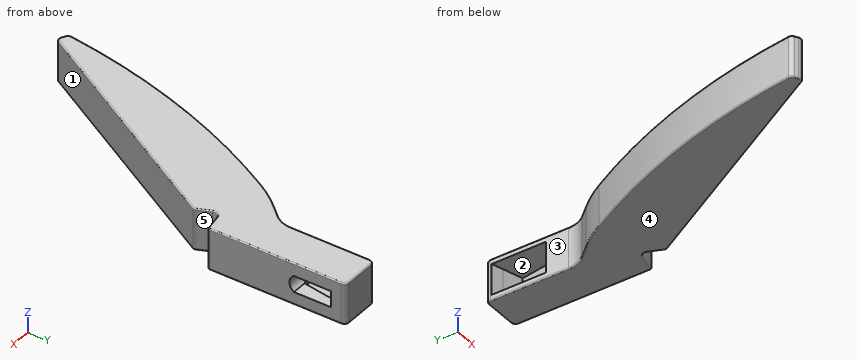
Autodesk Fusion 360 part; units mm, degrees
sketch "Sketch1" plane through (0, 0, 0) normal (1, 0, 0) x (0, 1, 0) in component "MitiVac Handle"
  line L0 (0, 0) -> (0, 3.5)
  line L1 (0, 3.5) -> (53.5, 3.5)
  line L2 (53.5, 3.5) -> (53.5, 0)
  line L3 (53.5, 0) -> (37.5, 0)
  line L4 (37.5, 0) -> (35.5, 0)
  line L5 (37.5, 0) -> (37.5, 3.5)
  line L6 (0, 0) -> (0, -3.5)
  line L7 (0, -3.5) -> (53.5, -3.5)
  line L8 (53.5, -3.5) -> (53.5, 0)
  line L9 (37.5, 0) -> (37.5, -3.5)
  arc A0 (37.5, 3.5) -> (37.5, -3.5) centre (39.5625, 0) ccw
  line L10 (0, 0) -> (53.5, 0)
  line L11 (0, 0) -> (53.5, 0)
  line L12 (0, 3.5) -> (0, 9)
  line L13 (0, -3.5) -> (0, -9)
  line L14 (0, 9) -> (30, 9)
  line L15 (30, 9) -> (30, 12.5)
  line L16 (30, 12.5) -> (60, 12.5)
  line L17 (60, 12.5) -> (60, 0)
  line L18 (0, -9) -> (30, -9)
  line L19 (30, -9) -> (30, -12.5)
  line L20 (30, -12.5) -> (60, -12.5)
  line L21 (60, -12.5) -> (60, 0)
  dimension "d1" = 3.5
  dimension "d2" = 53.5
  dimension "d3" = 3.5
  dimension "d4" = 16
  dimension "d5" = 2
  dimension "d6" = 3.5
  dimension "d7" = 53.5
  dimension "d8" = 5.5
  dimension "d9" = 5.5
  dimension "d10" = 30
  dimension "d11" = 3.5
  dimension "d12" = 30
  dimension "d13" = 12.5
  dimension "d14" = 30
  dimension "d15" = 3.5
  dimension "d16" = 30
sketch "Sketch2" plane through (0, 0, 0) normal (0, 0, 1) x (1, 0, 0) in component "MitiVac Handle"
  line L0 (0, 0) -> (0, 53.5)
  line L1 (0, 0) -> (-10.667, -1.6895)
  line L2 (0, 0) -> (9, 0) construction
  line L3 (-10.667, -1.6895) -> (-6.7597, -10.8945)
  line L4 (-10.667, -1.6895) -> (-0.667, -1.6895) construction
  line L5 (0, 0) -> (-6.7597, -10.8945)
  line L6 (-6.7597, -10.8945) -> (18.2403, -10.8945) construction
  line L7 (0, 0) -> (0, -40)
  line L8 (0, -40) -> (-63.5674, -110.5988)
  line L9 (0, -40) -> (95, -40) construction
  line L10 (-63.5674, -110.5988) -> (-6.7597, -10.8945)
  line L11 (0, 53.5) -> (0, 60)
  line L12 (0, 60) -> (-12.5, 60)
  line L13 (-12.5, 60) -> (-12.5, 25)
  line L14 (-63.5674, -110.5988) -> (-67.9117, -108.1235)
  line L15 (-10.667, -1.6895) -> (-28.7932, 6.7629)
  line L16 (-10.667, -1.6895) -> (9.333, -1.6895) construction
  line L17 (-28.7932, 6.7629) -> (-12.5, 25)
  line L18 (-28.7932, 6.7629) -> (-54.1503, -47.6156)
  arc A0 (-28.7932, 6.7629) -> (-67.9117, -108.1235) centre (217.624, -141.2447) ccw
  line L19 (0, 53.5) -> (-4, 53.5)
  line L20 (0, 53.5) -> (0, 37.5)
  line L21 (0, 37.5) -> (0, 35.5)
  line L22 (0, 37.5) -> (-6.5, 37.5)
  line L23 (-6.5, 37.5) -> (-4, 53.5)
  line L24 (-12.5, 60) -> (-12.5, 56)
  line L25 (-12.5, 56) -> (-4, 53.5)
  line L26 (-6.5, 37.5) -> (-12.5, 37.5)
  line L27 (-12.5, 37.5) -> (-12.5, 35.5)
  line L28 (-6.5, 37.5) -> (-12.5, 35.5)
  line L29 (-12.5, 60) -> (-17.5, 60)
  line L30 (-17.5, 60) -> (-17.5, 19.4035)
  line L31 (-12.5, 35.5) -> (-17.5, 33.8333)
  line L32 (-12.5, 56) -> (-17.5, 57.4706)
  dimension "d17" = 53.5
  dimension "d18" = 10.8
  dimension "d19" = 171
  dimension "d20" = 67
  dimension "d21" = 10
  dimension "d24" = 40
  dimension "d25" = 132
  dimension "d26" = 95
  dimension "d27" = 6.5
  dimension "d28" = 12.5
  dimension "d29" = 35
  dimension "d30" = 5
  dimension "d31" = 155
  dimension "d32" = 20
  dimension "d33" = 60
  dimension "d34" = 4
  dimension "d35" = 16
  dimension "d36" = 2
  dimension "d37" = 6.5
  dimension "d38" = 4
  dimension "d39" = 2
  dimension "d66" = 5
extrude "Extrude1" add sketch "Sketch2" along normal mid plane 18 contours L0 L1 L13 L15 L17 L21 L22 L28 | L3 L10 L14 L15 L18 A0 | L0 L19 L20 L22 L23 | L18 A0 | L11 L12 L13 L19 L24 L25 | L13 L23 L25 L26 | L13 L26 L27 L28 | L13 L17 L30 L31 | L13 L27 L30 L31 L32 | L13 L24 L29 L30 L32 in component "MitiVac Handle"
extrude "Extrude3" cut sketch "Sketch1" against normal up to surface (17.5 mm away) contours L4 L5 A0 L10 L11 | L4 L9 A0 L10 L11 | L1 L2 L3 L5 L10 L11 | L3 L7 L8 L9 L10 L11 in component "MitiVac Handle"
extrude "Extrude4" cut sketch "Sketch2" along normal mid plane 13.5 contours L13 L23 L25 L26 | L13 L26 L27 L28 | L13 L27 L30 L31 L32 in component "MitiVac Handle"
fillet "Fillet2" radius 2.5 1 edges at (-10.667, -1.6895, 0) in component "MitiVac Handle"
fillet "Fillet2" radius 1 2 edges at (0, 0, 0) (-6.7597, -10.8945, 0) in component "MitiVac Handle"
fillet "Fillet2" radius 2 2 edges at (0, 60, 0) (-17.5, 60, 0) in component "MitiVac Handle"
fillet "Fillet2" radius 12 1 edges at (-17.5, 19.4035, 0) in component "MitiVac Handle"
fillet "Fillet2" radius 65 1 edges at (-28.7932, 6.7629, 0) in component "MitiVac Handle"
fillet "Fillet2" radius 2 2 edges at (-67.9117, -108.1235, 0) (-63.5674, -110.5988, 0) in component "MitiVac Handle"
fillet "Fillet3" radius 0.5 2 faces at (-29.4988, -14.8978, 9) (-29.4988, -14.8978, -9) in component "MitiVac Handle"
component "MitiVac Handle" placed x (1, 0, 0) y (0, 1, 0) z (0, 0, 1) at (0, 0, 0)
equation "d3 = d1"
equation "d6 = d1"
equation "d7 = d2"
equation "d8 = ( 18 / 2 ) * 1 mm - 3.5 mm"
equation "d9 = d8"
equation "d11 = ( 25 / 2 ) * 1 mm - d8 - d1"
equation "d12 = 60 mm - d10"
equation "d13 = d11 + d8 + d1"
equation "d14 = d10"
equation "d15 = d11"
equation "d16 = d12"
equation "d19 = 180 deg - 9 deg"
equation "d25 = 270 deg - 138 deg"
equation "d46 = ( 13.5 / 2 ) * 1 mm"
Model file for the job. Use its own axes, mm. Face numbers are marked on the shaded views. A direction names the side the tool comes from. Give positions to 0.01 mm unless a question says otherwise; leave off trailing zeros. Loops run counter-clockwise (first coordinate to the right, second up) from the corner with the lowest first, then second, coordinate; pieces in that order, holes last. Notation, with made-up numbers: (69, 14) - (99, 14) arc R16 cw to (99, 18) - close; hole circle Ø4 at (53.5, 62.25). An arc over 180 degrees is marked (long way). One line per item, written item: value. Start each with the question number.
1. Slice it at A-A (z = 5). List the corners of the cut face in (x, y), plus the area to 3 significant figures.
2. Slice it at B-B (y = 40). List the corners of the cut face in (x, z).
3. Probe L1, parallel to X at y = 49.5, z = 3.75 (3 decimals); L2, parallel to Y at x = -10.5, z = 5.75; L3, parallel to Y at x = -17, z = 0. List the from-to ranges inside material, lowest first. Write a range as from..to.
4. Pull direction Y, two halves, no side cores. Call the marked faces 1, 2 and 3: pulls with the +Y half, pulls with the -Y half, needs draft (parallel to the pull), parting line crosses it, or undercut.
5. Pin check, flat tips, straight feed: pin 1 (1.2 mm diameter, centred on x = -1.5, z = 1.5, fed in from -Y); pin 2 (5 mm diameter, centred on x = -18.5, z = -7, fed in from +Y); pin 3 (1 mm diameter, centred on x = -36, z = 3.5, fed in from -Y). Stop position of each tip, or through.
6. Which spindle directions (+Z, -Z, +X, -X, +Y, -Y) get a long thin tool onto all of the face, cutting with end or side? Do the marked faces 4 and 5. Say none if no direction does.
Solution:
1. outline: (-67.76, -106.8) arc R2 ccw to (-66.76, -108.78) - (-65.31, -109.61) arc R2 ccw to (-62.58, -108.86) - (-7, -11.32) arc R1 ccw to (-6.95, -10.44) - (-9.42, -4.63) arc R2.5 cw to (-7.51, -1.19) - (-0.84, -0.13) arc R1 ccw to (0, 0.85) - (0, 58) arc R2 ccw to (-2, 60) - (-15.5, 60) arc R2 ccw to (-17.5, 58) - (-17.5, 57.47) - (-12.5, 56) - (-4, 53.5) - (-6.5, 37.5) - (-12.5, 35.5) - (-17.5, 33.83) - (-17.5, 23.98) arc R12 cw to (-20.55, 15.99) - (-24.44, 11.64) arc R65 ccw to (-32.53, 0.35) arc R287.45 ccw to start
1. area: 3,410 mm^2
2. outline: (-17.5, -8.5) arc R0.5 ccw to (-17, -9) - (-0.5, -9) arc R0.5 ccw to (0, -8.5) - (0, -3.5) - (-6.11, -3.5) - (-6.11, -6.75) - (-17.5, -6.75) - close; (-17.5, 6.75) - (-6.11, 6.75) - (-6.11, 3.5) - (0, 3.5) - (0, 8.5) arc R0.5 ccw to (-0.5, 9) - (-17, 9) arc R0.5 ccw to (-17.5, 8.5) - close
3. L1: x = -4.625..0
3. L2: y = -17.46..36.17, 55.41..60
3. L3: y = -28.87..34, 57.32..59.32
4. face 1: pulls with the -Y half
4. face 2: undercut
4. face 3: needs draft
5. pin 1: stops at y = -0.33
5. pin 2: stops at y = 59.94
5. pin 3: stops at y = -63.09
6. face 4: -Z, +X, -X, +Y, -Y
6. face 5: +Z, -Z, +X
